Verification items for the finished model (mm, model axes). Face numbers are marked on the shaded views. Round coordinates to 2 decimals unless told otherwise and drop trailing zeros. Loops run counter-clockwise (first coordinate to the right, second up) from the corner with the lowest first, then second, coordinate; pieces in that order, holes last. Notation, with made-up numbers: M 13,64.5 L 33,64.5 A17 ccw 33,72.5 Z; hole C 33.25,74.5 d10. An arc over 180 degrees is marked long. Answer as CSV lines item,"result".
```python
from build123d import *

# Parameters (mm, degrees)
CROQUIS1_W              = 44
CROQUIS1_H              = 44
CROQUIS1_R              = 11.5
SALIENTE_EXTRUIR1_DEPTH = 10
CROQUIS2_R              = 1.75
CORTAR_EXTRUIR1_DEPTH   = 33.680269277
REDONDEO1_R             = 2


with BuildPart() as part:
    # Croquis1 → Saliente-Extruir1 (new body)
    with BuildSketch(Plane(origin=(0, 0, 0), x_dir=(1, 0, 0), z_dir=(0, 1, 0))):
        Rectangle(CROQUIS1_W, CROQUIS1_H)
        with Locations(Location((0, 0, 0), (0, 0, 270))):
            Circle(CROQUIS1_R, mode=Mode.SUBTRACT)
    extrude(amount=SALIENTE_EXTRUIR1_DEPTH)

    # Croquis2 → Cortar-Extruir1 (cut, through all)
    with BuildSketch(Plane(origin=(0, 10, 0), x_dir=(1, 0, 0), z_dir=(0, 1, 0))):
        with Locations(Location((0, 16.88, 0), (0, 0, 270))):
            Circle(CROQUIS2_R)
        with Locations(Location((0, -16.88, 0), (0, 0, 270))):
            Circle(CROQUIS2_R)
    extrude(amount=-CORTAR_EXTRUIR1_DEPTH, mode=Mode.SUBTRACT)

    # Redondeo1
    redondeo1_edges = [part.edges().sort_by_distance(p)[0] for p in [
        (22, 5, 22),
        (-22, 5, 22),
        (-22, 5, -22),
        (22, 5, -22),
    ]]
    fillet(redondeo1_edges, radius=REDONDEO1_R)


solid = part.part
```
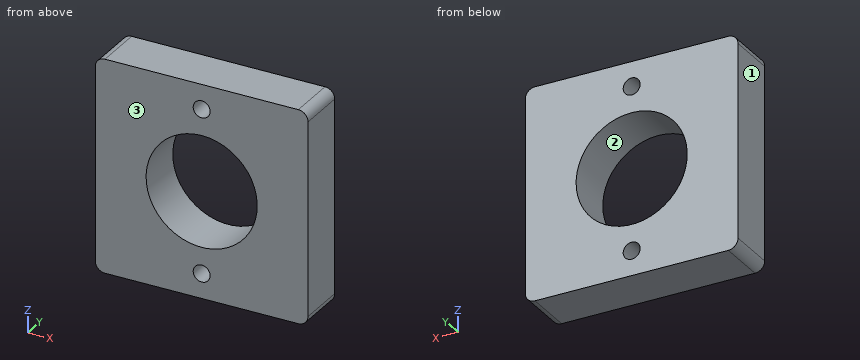
1) Section check B-B (y = 0.75). Record the cut outline in (x, z).
Here are the results:
outline,"M -22,-20 A2 ccw -20,-22 L 20,-22 A2 ccw 22,-20 L 22,20 A2 ccw 20,22 L -20,22 A2 ccw -22,20 Z; hole C 0,0 d23; hole C 0,-16.88 d3.5; hole C 0,16.88 d3.5"
2) Section check C-C (z = -16.88). Record the cut outline in (x, y), plus the area to 3 significant figures.
Here are the results:
outline,"M -22,0 L -1.75,0 L -1.75,10 L -22,10 Z; M 1.75,0 L 22,0 L 22,10 L 1.75,10 Z"
area,"405 mm^2"
3) Section check D-D (z = 0). Record the cut outline in (x, y).
Here are the results:
outline,"M -22,0 L -11.5,0 L -11.5,10 L -22,10 Z; M 11.5,0 L 22,0 L 22,10 L 11.5,10 Z"
4) Material ranges on probe 1 along X at (y, z) = (1.5, 17); probe 2 along X at (y, z) = (6.25, 0); probe 3 along Z at (x, y) = (2.5, 7.5), recorded low to high.
Here are the results:
probe 1,"x = -22 to -1.75, 1.75 to 22"
probe 2,"x = -22 to -11.5, 11.5 to 22"
probe 3,"z = -22 to -11.22, 11.22 to 22"
5) Section check A-A (x = 0). Record the cut outline in (y, z), plus the area to 3 significant figures.
Here are the results:
outline,"M 0,-22 L 10,-22 L 10,-18.63 L 0,-18.63 Z; M 0,-15.13 L 10,-15.13 L 10,-11.5 L 0,-11.5 Z; M 0,11.5 L 10,11.5 L 10,15.13 L 0,15.13 Z; M 0,18.63 L 10,18.63 L 10,22 L 0,22 Z"
area,"140 mm^2"
6) Draft check along X on the marked faces 1, 2 and 3. Enter one of: +X half, -X half, draft (parallel to the pull), parting line (faces both ways), or undercut.
Here are the results:
face 1,"-X half"
face 2,"undercut"
face 3,"draft"
